from build123d import *

# Parameters (mm, degrees)
SKETCH1_R           = 6.35
BOSS_EXTRUDE1_DEPTH = 62.3062
SKETCH2_W           = 25.005940549
SKETCH2_H           = 0.9906
SKETCH3_W           = 23.546175461
SKETCH3_H           = 0.9906
SKETCH4_W           = 18.658380353
SKETCH4_H           = 0.9906
SKETCH5_W           = 21.890491914
SKETCH5_H           = 0.9906
CUT_EXTRUDE1_DEPTH  = 1.778
CUT_EXTRUDE2_DEPTH  = 1.778


with BuildPart() as part:
    # Sketch1 → Boss-Extrude1 (new body)
    with BuildSketch(Plane(origin=(0, 0, 0), x_dir=(1, 0, 0), z_dir=(0, 1, 0))):
        Circle(SKETCH1_R)
    extrude(amount=BOSS_EXTRUDE1_DEPTH)

    # Sketch2 → Cut-Revolve1 (revolve, cut)
    with BuildSketch(Plane(origin=(0, 0, 0), x_dir=(0, 0, -1), z_dir=(1, 0, 0))):
        with Locations((-18.446570275, 52.2859)):
            Rectangle(SKETCH2_W, SKETCH2_H)
    revolve(axis=Axis((0, 57.347973558, 0), (0, -1, 0)), mode=Mode.SUBTRACT)

    # Sketch3 → Cut-Revolve2 (revolve, cut)
    with BuildSketch(Plane(origin=(0, 0, 0), x_dir=(0, 0, -1), z_dir=(1, 0, 0))):
        with Locations((-17.71668773, 38.5953)):
            Rectangle(SKETCH3_W, SKETCH3_H)
    revolve(axis=Axis((0, 44.893049612, 0), (0, -1, 0)), mode=Mode.SUBTRACT)

    # Sketch4 → Cut-Revolve3 (revolve, cut)
    with BuildSketch(Plane(origin=(0, 0, 0), x_dir=(0, 0, -1), z_dir=(1, 0, 0))):
        with Locations((-15.272790177, 30.0609)):
            Rectangle(SKETCH4_W, SKETCH4_H)
    revolve(axis=Axis((0, 32.886405358, 0), (0, -1, 0)), mode=Mode.SUBTRACT)

    # Sketch5 → Cut-Revolve4 (revolve, cut)
    with BuildSketch(Plane(origin=(0, 0, 0), x_dir=(0, 0, -1), z_dir=(1, 0, 0))):
        with Locations((-16.888845957, 10.0203)):
            Rectangle(SKETCH5_W, SKETCH5_H)
    revolve(axis=Axis((0, 12.888921404, 0), (0, -1, 0)), mode=Mode.SUBTRACT)

    # Sketch6 → Cut-Extrude1 (cut)
    with BuildSketch(Plane(origin=(6.35, 0, 0), x_dir=(0, 0, -1), z_dir=(1, 0, 0))):
        with BuildLine():
            Line((1.5875, 51.7906), (1.5875, 39.0906))
            ThreePointArc((1.5875, 39.0906), (0, 37.5031), (-1.5875, 39.0906))
            Line((-1.5875, 39.0906), (-1.5875, 51.7906))
            ThreePointArc((-1.5875, 51.7906), (0, 53.3781), (1.5875, 51.7906))
        make_face()
    extrude(amount=-CUT_EXTRUDE1_DEPTH, mode=Mode.SUBTRACT)

    # Sketch7 → Cut-Extrude2 (cut)
    with BuildSketch(Plane(origin=(6.35, 0, 0), x_dir=(0, 0, -1), z_dir=(1, 0, 0))):
        with BuildLine():
            Line((1.5875, 29.5656), (1.5875, 10.5156))
            ThreePointArc((1.5875, 10.5156), (0, 8.9281), (-1.5875, 10.5156))
            Line((-1.5875, 10.5156), (-1.5875, 29.5656))
            ThreePointArc((-1.5875, 29.5656), (0, 31.1531), (1.5875, 29.5656))
        make_face()
    extrude(amount=-CUT_EXTRUDE2_DEPTH, mode=Mode.SUBTRACT)


solid = part.part
The listing builds one solid part. Answer for the finished solid, in the listing's coordinates (mm). A direction names the side the tool comes from. Round coordinates to 2 decimals unless told otherwise and drop trailing zeros. Order: outer loops, then holes, each group sorted by start corner. A loop starts at its lowest first (then second) coordinate and runs counter-clockwise, first axis right, second up. Notation, with made-up numbers: M -10,-35.75 L 45,-35.75 A32 cw 45,-5.75 Z; hole C 56.25,85.25 d5. An arc over 180 degrees is marked long. Answer in a Markdown table with one row per item. Add a question column.
1) Consider line 1 along Z through (x, y) = (-0.25, 20); line 2 along Z through (x, y) = (5, 48.5); line 3 along Z through (x, y) = (5.25, 41). Determine where each line is inside the solid, lowest interval first. Write a range as from..to.
2) The part is cut by section A-A on z = 0. Determine the outline of the cut face in (x, y) (3 decimals), plus the area to 3 significant figures.
3) Determine the mould class of faces 4 (the face through (0, 62.306, 0)), 5 (the face through (-6.345, 19.907, -0.257)), 6 (the face through (5, 46, -1.588)) for opening direction Y: pulls with the +Y half, pulls with the -Y half, needs draft (parallel to the pull), parting line crosses it, or undercut.
4) The part is cut by section B-B on y = 18. Determine the outline of the cut face in (x, z).
5) Which of the six approach directions +Z, -Z, +X, -X, +Y, -Y give full straight-line access (tool end or side, diameter ignored) to faces 1 (the face through (-6.1, 52.781, 0)), 2 (the face through (5.276, 37.503, -0.035)), 3 (the face through (-6.345, 45.352, -0.257))?
6) Flat-ended cylindrical pins translate along their axes: pin 1 Ø0.8 at (x, y) = (5, 24.5) entering from -Z; pin 2 Ø4 at (y, z) = (27, 2.5) entering from -X; pin 3 Ø3 at (x, z) = (-5, 2) entering from -Y; pin 4 Ø1.6 at (y, z) = (42.5, 0) entering from +X. Find the tip coordinate at first contact, or state that the pin passes through.
Findings below:
| question | item | result |
|---|---|---|
| 1 | line 1 | z = -6.35..6.35 |
| 1 | line 2 | z = -3.91..-1.59, 1.59..3.91 |
| 1 | line 3 | z = -3.57..-1.59, 1.59..3.57 |
| 2 | outline | M -6.35,0 L 6.35,0 L 6.35,8.928 L 4.572,8.928 L 4.572,31.153 L 6.35,31.153 L 6.35,37.503 L 4.572,37.503 L 4.572,53.378 L 6.35,53.378 L 6.35,62.306 L -6.35,62.306 L -6.35,52.781 L -5.944,52.781 L -5.944,51.791 L -6.35,51.791 L -6.35,39.091 L -5.944,39.091 L -5.944,38.1 L -6.35,38.1 L -6.35,30.556 L -5.944,30.556 L -5.944,29.566 L -6.35,29.566 L -6.35,10.516 L -5.944,10.516 L -5.944,9.525 L -6.35,9.525 Z |
| 2 | area | 722 mm² |
| 3 | face 4 | pulls with the +Y half |
| 3 | face 5 | needs draft |
| 3 | face 6 | undercut |
| 4 | outline | M 4.57,-1.59 L 4.57,1.59 L 6.15,1.59 A6.35 ccw long 6.15,-1.59 Z |
| 5 | face 1 | none |
| 5 | face 2 | +X |
| 5 | face 3 | +Y, -Y |
| 6 | pin 1 | stops at z = -4.38 |
| 6 | pin 2 | stops at x = -6.33 |
| 6 | pin 3 | stops at y = 0 |
| 6 | pin 4 | stops at x = 4.57 |
